from build123d import *

# Parameters (mm, degrees)
BOSS_EXTRUDE1_DEPTH = 6.35


with BuildPart() as part:
    # Model → Boss-Extrude1 (new body)
    with BuildSketch(Plane.XY):
        with BuildLine():
            Line((151.543552764, 90.714118443), (4.731109074, 179.975171138))
            ThreePointArc((4.731109074, 179.975171138), (-4.6204e-05, 189.797926504), (7.04414309, 198.119569997))
            ThreePointArc((7.04414309, 198.119569997), (64.007829995, 241.277120886), (104.121959965, 300.423485114))
            ThreePointArc((104.121959965, 300.423485114), (133.652754943, 444.147036942), (126.82389853, 590.714065711))
            ThreePointArc((126.82389853, 590.714065711), (96.817440989, 786.388398141), (87.971677303, 984.152359294))
            ThreePointArc((87.971677303, 984.152359294), (81.447636866, 1031.694941858), (59.670586387, 1074.457312383))
            ThreePointArc((59.670586387, 1074.457312383), (58.804071749, 1079.18754246), (60.242621079, 1083.776278673))
            ThreePointArc((60.242621079, 1083.776278673), (63.654473657, 1087.165258783), (68.252782173, 1088.572910369))
            ThreePointArc((68.252782173, 1088.572910369), (116.239658622, 1088.919247204), (161.450686905, 1105.007229742))
            ThreePointArc((161.450686905, 1105.007229742), (341.097480319, 1188.168888466), (528.627670124, 1251.582292231))
            ThreePointArc((528.627670124, 1251.582292231), (638.840136142, 1299.353501718), (737.100152906, 1368.446520373))
            ThreePointArc((737.100152906, 1368.446520373), (756.919068228, 1386.450533813), (775.901150633, 1405.334772002))
            ThreePointArc((775.901150633, 1405.334772002), (809.950243775, 1468.168640901), (822.049885165, 1538.603252442))
            ThreePointArc((822.049885165, 1538.603252442), (824.185406932, 1546.845116579), (831.891796136, 1550.464556193))
            Line((831.891796136, 1550.464556193), (914.542928671, 1550.464556193))
            Line((914.542928671, 1550.464556193), (997.194061205, 1550.464556193))
            ThreePointArc((997.194061205, 1550.464556193), (1004.900450409, 1546.845116579), (1007.035972176, 1538.603252442))
            ThreePointArc((1007.035972176, 1538.603252442), (1019.135613566, 1468.168640901), (1053.184706708, 1405.334772002))
            ThreePointArc((1053.184706708, 1405.334772002), (1072.166789113, 1386.450533813), (1091.985704435, 1368.446520373))
            ThreePointArc((1091.985704435, 1368.446520373), (1190.245721199, 1299.353501718), (1300.458187217, 1251.582292231))
            ThreePointArc((1300.458187217, 1251.582292231), (1487.988377024, 1188.168888466), (1667.635170438, 1105.00722974))
            ThreePointArc((1667.635170438, 1105.00722974), (1712.84619872, 1088.919247204), (1760.833075168, 1088.572910369))
            ThreePointArc((1760.833075168, 1088.572910369), (1765.431383684, 1087.165258783), (1768.843236262, 1083.776278673))
            ThreePointArc((1768.843236262, 1083.776278673), (1770.281785592, 1079.18754246), (1769.415270954, 1074.457312383))
            ThreePointArc((1769.415270954, 1074.457312383), (1747.638220475, 1031.694941858), (1741.114180038, 984.152359294))
            ThreePointArc((1741.114180038, 984.152359294), (1732.268416352, 786.388398141), (1702.261958811, 590.714065711))
            ThreePointArc((1702.261958811, 590.714065711), (1695.433102398, 444.147036942), (1724.963897376, 300.423485114))
            ThreePointArc((1724.963897376, 300.423485114), (1765.078027346, 241.277120886), (1822.041714251, 198.119569997))
            ThreePointArc((1822.041714251, 198.119569997), (1829.085903545, 189.797926504), (1824.354748267, 179.975171138))
            Line((1824.354748267, 179.975171138), (1677.542304577, 90.714118443))
            Line((1677.542304577, 90.714118443), (1530.729860887, 1.453065748))
            ThreePointArc((1530.729860887, 1.453065748), (1519.831798271, 1.773353837), (1515.685681443, 11.857007366))
            ThreePointArc((1515.685681443, 11.857007366), (1503.586040054, 82.291618906), (1469.536946912, 145.125487805))
            ThreePointArc((1469.536946912, 145.125487805), (1450.554864506, 164.009725995), (1430.735949184, 182.013739434))
            ThreePointArc((1430.735949184, 182.013739434), (1332.475932423, 251.106758088), (1222.26346641, 298.877967574))
            ThreePointArc((1222.26346641, 298.877967574), (1106.620134686, 335.316646956), (993.62301558, 379.280366099))
            ThreePointArc((993.62301558, 379.280366099), (954.903308451, 391.364362796), (914.542928671, 395.39901772))
            ThreePointArc((914.542928671, 395.39901772), (874.182548891, 391.364362796), (835.462841761, 379.280366099))
            ThreePointArc((835.462841761, 379.280366099), (722.465722657, 335.316646957), (606.822390935, 298.877967575))
            ThreePointArc((606.822390935, 298.877967575), (496.609924919, 251.106758089), (398.349908157, 182.013739434))
            ThreePointArc((398.349908157, 182.013739434), (378.530992835, 164.009725995), (359.548910429, 145.125487805))
            ThreePointArc((359.548910429, 145.125487805), (325.499817287, 82.291618906), (313.400175898, 11.857007366))
            ThreePointArc((313.400175898, 11.857007366), (309.25405907, 1.773353837), (298.355996454, 1.453065748))
            Line((298.355996454, 1.453065748), (151.543552764, 90.714118443))
        make_face()
        with BuildLine():
            Line((193.777874867, 221.294540203), (228.097625685, 277.742076191))
            ThreePointArc((228.097625685, 277.742076191), (267.717827548, 382.549812212), (266.789374301, 494.592482209))
            ThreePointArc((266.789374301, 494.592482209), (241.770965978, 627.59734054), (218.673506786, 760.949207694))
            ThreePointArc((218.673506786, 760.949207694), (218.167687021, 829.167165589), (232.404753167, 895.884866243))
            ThreePointArc((232.404753167, 895.884866243), (231.841152746, 929.369079724), (210.559765814, 955.226627329))
            Line((210.559765814, 955.226627329), (204.638979738, 958.826428441))
            ThreePointArc((204.638979738, 958.826428441), (194.004142064, 1002.450105815), (237.627819438, 1013.084943489))
            Line((237.627819438, 1013.084943489), (243.548605514, 1009.485142378))
            ThreePointArc((243.548605514, 1009.485142378), (276.299184629, 1002.491590666), (306.286010429, 1017.401335007))
            ThreePointArc((306.286010429, 1017.401335007), (358.96611995, 1060.745904377), (419.763138988, 1091.692117541))
            ThreePointArc((419.763138988, 1091.692117541), (595.228682895, 1146.768807529), (771.739960804, 1198.39600627))
            ThreePointArc((771.739960804, 1198.39600627), (851.898170732, 1253.089548855), (882.79292867, 1345.079962222))
            Line((882.79292867, 1345.079962222), (882.79292867, 1345.660139454))
            ThreePointArc((882.79292867, 1345.660139454), (892.092288368, 1368.110779757), (914.542928671, 1377.410139455))
            ThreePointArc((914.542928671, 1377.410139455), (936.993568973, 1368.110779757), (946.292928671, 1345.660139454))
            Line((946.292928671, 1345.660139454), (946.292928671, 1345.079962222))
            ThreePointArc((946.292928671, 1345.079962222), (977.187686609, 1253.089548855), (1057.345896537, 1198.39600627))
            ThreePointArc((1057.345896537, 1198.39600627), (1233.857174446, 1146.768807529), (1409.322718353, 1091.692117541))
            ThreePointArc((1409.322718353, 1091.692117541), (1470.119737391, 1060.745904377), (1522.799846912, 1017.401335006))
            ThreePointArc((1522.799846912, 1017.401335006), (1552.786672713, 1002.491590666), (1585.537251828, 1009.485142378))
            Line((1585.537251828, 1009.485142378), (1591.458037903, 1013.084943489))
            ThreePointArc((1591.458037903, 1013.084943489), (1635.081715277, 1002.450105815), (1624.446877603, 958.826428441))
            Line((1624.446877603, 958.826428441), (1618.526091527, 955.226627329))
            ThreePointArc((1618.526091527, 955.226627329), (1597.244704595, 929.369079725), (1596.681104174, 895.884866243))
            ThreePointArc((1596.681104174, 895.884866243), (1610.91817032, 829.167165589), (1610.412350555, 760.949207694))
            ThreePointArc((1610.412350555, 760.949207694), (1587.314891364, 627.597340544), (1562.296483041, 494.592482218))
            ThreePointArc((1562.296483041, 494.592482218), (1561.368029793, 382.549812216), (1600.988231656, 277.742076191))
            Line((1600.988231656, 277.742076191), (1635.307982474, 221.294540203))
            ThreePointArc((1635.307982474, 221.294540203), (1624.673144799, 177.670862829), (1581.049467425, 188.305700503))
            Line((1581.049467425, 188.305700503), (1546.729716607, 244.753236491))
            ThreePointArc((1546.729716607, 244.753236491), (1471.914922649, 328.162879411), (1372.015609312, 378.902894406))
            ThreePointArc((1372.015609312, 378.902894406), (1242.41928054, 417.90295417), (1113.398935267, 458.768142267))
            ThreePointArc((1113.398935267, 458.768142267), (1039.69925486, 497.387302002), (993.069617081, 566.298543982))
            ThreePointArc((993.069617081, 566.298543982), (988.420625683, 572.364700977), (981.132076965, 574.664361651))
            Line((981.132076965, 574.664361651), (959.146552953, 574.664361651))
            ThreePointArc((959.146552953, 574.664361651), (950.426671687, 571.197653085), (946.467308072, 562.690136563))
            ThreePointArc((946.467308072, 562.690136563), (936.486383713, 541.343696224), (914.542586541, 532.755382542))
            ThreePointArc((914.542586541, 532.755382542), (892.599225651, 541.343933359), (882.618549269, 562.690136563))
            ThreePointArc((882.618549269, 562.690136563), (878.659185654, 571.197653084), (869.939304388, 574.664361651))
            Line((869.939304388, 574.664361651), (847.953780376, 574.664361651))
            ThreePointArc((847.953780376, 574.664361651), (840.66523167, 572.364700961), (836.01624026, 566.298543983))
            ThreePointArc((836.01624026, 566.298543983), (789.386602481, 497.387302002), (715.686922074, 458.768142267))
            ThreePointArc((715.686922074, 458.768142267), (586.666576793, 417.902954168), (457.070248014, 378.902894401))
            ThreePointArc((457.070248014, 378.902894401), (357.170934686, 328.162879406), (282.356140734, 244.753236492))
            Line((282.356140734, 244.753236492), (248.036389916, 188.305700503))
            ThreePointArc((248.036389916, 188.305700503), (204.412712542, 177.670862829), (193.777874867, 221.294540203))
        make_face(mode=Mode.SUBTRACT)
    extrude(amount=BOSS_EXTRUDE1_DEPTH)


solid = part.part
Check sheet for the modelled part. Datum: model origin and axes. Units: mm. A direction names the side the tool comes from. Round coordinates to 2 decimals unless told otherwise and drop trailing zeros. Loops run counter-clockwise (first coordinate to the right, second up) from the corner with the lowest first, then second, coordinate; pieces in that order, holes last. Notation, with made-up numbers: (4, 73) -> (28, 73) arc R17 cw to (28, 91) -> close; hole circle Ø6 at (-15.5, -32.75). An arc over 180 degrees is marked (long way). Put each result on its own line as item: value. Start each with the question number.
1. Section check C-C (y = 1442). Enter the section's corners in (x, z), plus the area to 3 significant figures.
2. Section check A-A (y = 818). Enter the section's corners in (x, z).
3. Gauge pin test, flat ends, axial feed: pin 1 (1 mm diameter, centred on y = 383, z = 4, fed in from -X); pin 2 (0.5 mm diameter, centred on y = 1345.5, z = 2, fed in from +X); pin 3 (0.5 mm diameter, centred on y = 1345.5, z = 3, fed in from -X). Record the tip position at first contact, or that the pin passes through.
4. Access from +Z, -Z, +X, -X, +Y, -Y to the whole of each face (thin tool, end or side, straight path). Record for faces 1 (the face through (1485.4, 1189.2, 3.1)), 2 (the face through (1503.913, 81.341, 3.131)), 3 (the face through (976.358, 1254.196, 3.131)).
5. Section check B-B (x = 693). Enter the section's corners in (y, z), plus the area to 3 significant figures.
6. Scan lines: probe 1 along Y at (x, z) = (212, 2); probe 2 along Y at (x, z) = (1621, 0.5); probe 3 along X at (y, z) = (666, 2.5). Record each from-to range of solid material in increasing order.
7. Draft check along Y on faces 4 (the face through (338.523, 1187.139, 3.131)), 5 (the face through (851.06, 1251.99, 3.13)), 6 (the face through (325.83, 83.24, 3.13)), 7 (the face through (592.76, 1146.02, 3.13)). Enter one of: +Y half, -Y half, draft (parallel to the pull), parting line (faces both ways), or undercut.
Findings:
1. outline: (798.95, 0) -> (1030.14, 0) -> (1030.14, 6.35) -> (798.95, 6.35) -> close
1. area: 1,470 mm^2
2. outline: (93.97, 0) -> (217.23, 0) -> (217.23, 6.35) -> (93.97, 6.35) -> close; (1611.85, 0) -> (1735.12, 0) -> (1735.12, 6.35) -> (1611.85, 6.35) -> close
3. pin 1: stops at x = 125.55
3. pin 2: stops at x = 1120.46
3. pin 3: stops at x = 708.63
4. face 1: +Z, -Z, +X, +Y
4. face 2: +Z, -Z, -Y
4. face 3: +Z, -Z
5. outline: (325.23, 0) -> (451.43, 0) -> (451.43, 6.35) -> (325.23, 6.35) -> close; (1175.83, 0) -> (1333.71, 0) -> (1333.71, 6.35) -> (1175.83, 6.35) -> close
5. area: 1,800 mm^2
6. probe 1: y = 53.96 to 174.33, 251.27 to 954.32, 1016.36 to 1130.8
6. probe 2: y = 56.34 to 175.75, 244.83 to 956.73, 1014.9 to 1128.88
6. probe 3: x = 112.73 to 234.92, 1594.17 to 1716.36
7. face 4: +Y half
7. face 5: undercut
7. face 6: -Y half
7. face 7: undercut
